Geometry check sheet. Reference: the model listing, model coordinates, mm. A direction names the side the tool comes from. Give positions to 0.01 mm unless a question says otherwise; leave off trailing zeros. Loops run counter-clockwise (first coordinate to the right, second up) from the corner with the lowest first, then second, coordinate; pieces in that order, holes last. Notation, with made-up numbers: (23, 51.25) -> (51, 51.25) arc R30 cw to (51, 80.25) -> close; hole circle Ø3 at (2.5, 5). An arc over 180 degrees is marked (long way). One line per question, with ' | ' between items.
from build123d import *

# Parameters (mm, degrees)
SKETCH_1_W          = 50
SKETCH_1_H          = 35
EXTRUDE_1_DEPTH     = 250
SKETCH_2_W          = 50
SKETCH_2_H          = 25
CUT_EXTRUDE_1_DEPTH = 240
CUT_EXTRUDE_2_DEPTH = 11
SKETCH_5_W          = 50
SKETCH_5_H          = 55
EXTRUDE_2_DEPTH     = 15


with BuildPart() as part:
    # 草图1 → 凸台-拉伸1 (new body)
    with BuildSketch(Plane(origin=(0, 0, 0), x_dir=(1, 0, 0), z_dir=(0, 1, 0))):
        Rectangle(SKETCH_1_W, SKETCH_1_H)
    extrude(amount=EXTRUDE_1_DEPTH)

    # 草图2 → 切除-拉伸1 (cut)
    with BuildSketch(Plane(origin=(0, 250, 0), x_dir=(1, 0, 0), z_dir=(0, 1, 0))):
        with Locations((0, 5)):
            Rectangle(SKETCH_2_W, SKETCH_2_H)
    extrude(amount=-CUT_EXTRUDE_1_DEPTH, mode=Mode.SUBTRACT)

    # 草图3 → 切除-拉伸2 (cut, through all)
    with BuildSketch(Plane(origin=(0, 10, 0), x_dir=(1, 0, 0), z_dir=(0, 1, 0))):
        with BuildLine():
            Line((-20.7, 1.5), (-20.7, 9.5))
            ThreePointArc((-20.7, 9.5), (-17.5, 12.7), (-14.3, 9.5))
            Line((-14.3, 9.5), (-14.3, 1.5))
            ThreePointArc((-14.3, 1.5), (-17.5, -1.7), (-20.7, 1.5))
        make_face()
        with BuildLine():
            Line((20.7, 1.5), (20.7, 9.5))
            ThreePointArc((20.7, 9.5), (17.5, 12.7), (14.3, 9.5))
            Line((14.3, 9.5), (14.3, 1.5))
            ThreePointArc((14.3, 1.5), (17.5, -1.7), (20.7, 1.5))
        make_face()
    extrude(amount=-CUT_EXTRUDE_2_DEPTH, mode=Mode.SUBTRACT)

    # 草图5 → 凸台-拉伸2 (add)
    with BuildSketch(Plane.XY.offset(17.5)):
        with Locations((0, 222.5)):
            Rectangle(SKETCH_5_W, SKETCH_5_H)
    extrude(amount=EXTRUDE_2_DEPTH)


solid = part.part
Item 1: Sectioned sample at B-B (z = -4). Record the cut outline in (x, y), plus the area to 3 significant figures.
Result:
outline: (-25, 0) -> (-20.7, 0) -> (-20.7, 10) -> (-25, 10) -> close; (-14.3, 0) -> (14.3, 0) -> (14.3, 10) -> (-14.3, 10) -> close; (20.7, 0) -> (25, 0) -> (25, 10) -> (20.7, 10) -> close | area: 372 mm2
Item 2: Sectioned sample at A-A (x = -17.5). Record the cut outline in (y, z), plus the area to 3 significant figures.
Result:
outline: (0, -17.5) -> (10, -17.5) -> (10, -12.7) -> (0, -12.7) -> close; (0, 1.7) -> (10, 1.7) -> (10, 7.5) -> (250, 7.5) -> (250, 32.5) -> (195, 32.5) -> (195, 17.5) -> (0, 17.5) -> close | area: 3,430 mm2
Item 3: Sectioned sample at C-C (y = 166.5). Record the cut outline in (x, z).
Result:
outline: (-25, 7.5) -> (25, 7.5) -> (25, 17.5) -> (-25, 17.5) -> close
Item 4: Scan lines: probe 1 along Y at (x, z) = (22, 27); probe 2 along Z at (x, y) = (-3, 156); probe 3 along Y at (x, z) = (5.5, -8.5). Record each from-to range of solid material in increasing order.
Result:
probe 1: 195 to 250 | probe 2: 7.5 to 17.5 | probe 3: 0 to 10
Item 5: Depth check by flat-ended pin: pin 1 Ø25 at (x, y) = (-0.5, 60) entering from +Z; pin 2 Ø6 at (x, z) = (14, -2.5) entering from +Y; pin 3 Ø7.5 at (x, z) = (1, 24.5) entering from -Y. Enter the tip coordinate at first touch or a pass-through.
Result:
pin 1: z = 17.5 | pin 2: y = 10 | pin 3: y = 195
Item 6: Release check for a two-part mould opening along X. For faces 1 (the face through (17.4, 5.1, 1.7)), 2 (the face through (0, 195, 25)), 3 (the face through (-25, 143, 15)) record: pulls with the +X half, pulls with the -X half, needs draft (parallel to the pull), parting line crosses it, or undercut.
Result:
face 1: undercut | face 2: needs draft | face 3: pulls with the -X half
Item 7: Set-up check for faces 4 (the face through (0, 96, 17.5)), 5 (the face through (-17.6, 5.1, -12.7)), 6 (the face through (0, 223, 32.5)), 7 (the face through (0, 0, 0)), 8 (the face through (0, 132, 7.5)): record each of +Z, -Z, +X, -X, +Y, -Y from which the full face is reachable in a straight line by a thin tool's end or side.
Result:
face 4: +Z, +X, -X, -Y | face 5: +Y, -Y | face 6: +Z, +X, -X, +Y, -Y | face 7: +Z, -Z, +X, -X, -Y | face 8: -Z, +X, -X, +Y
Item 8: Sectioned sample at D-D (x = 18). Record the cut outline in (y, z), plus the area to 3 significant figures.
Result:
outline: (0, -17.5) -> (10, -17.5) -> (10, -12.66) -> (0, -12.66) -> close; (0, 1.66) -> (10, 1.66) -> (10, 7.5) -> (250, 7.5) -> (250, 32.5) -> (195, 32.5) -> (195, 17.5) -> (0, 17.5) -> close | area: 3,430 mm2
